Check sheet for the modelled part. Datum: model origin and axes. Units: mm. A direction names the side the tool comes from. Give positions to 0.01 mm unless a question says otherwise; leave off trailing zeros. Write each loop counter-clockwise with the first axis right and the second up, starting at its lowest first coordinate (ties: lowest second). Pieces come first, ordered by that corner, then holes. Notation, with made-up numbers: (-9, -36.75) -> (37, -36.75) arc R19 cw to (37, -11.75) -> close; hole circle Ø11 at (-32.5, 21.25). An arc over 180 degrees is marked (long way). Use a Markdown table: item, result. Add a question column.
1. Cross-section at D-D (z = 27). Enter the section's corners in (x, y), then the cut area to 3 significant figures.
2. Cross-section at B-B (z = 54). Enter the section's corners in (x, y), then the cut area to 3 significant figures.
3. Release check for a two-part mould opening along X. For faces 1 (the cylindrical face through (12.675, 34.614, 48.128)), 2 (the flat face through (180, 30, 12)), 3 (the cylindrical face through (52.017, 30.791, 12.675)) record: released by +X, released by -X, zero draft, split by the parting line, or undercut.
4. Cross-section at A-A (x = 70). Enter the section's corners in (y, z), then the cut area to 3 significant figures.
5. Cross-section at C-C (y = 26). Enter the section's corners in (x, z), then the cut area to 3 significant figures.
6. Set-up check for faces 4 (the flat face through (101, 30, 25)), 5 (the cylindrical face through (12.675, 8.555, 77.979)): record each of +Z, -Z, +X, -X, +Y, -Y from which the full face is reachable in a straight line by a thin tool's end or side.
7. Gauge pin test, flat ends, axial feed: P1, Ø3, axis at y = 31.5, z = 43, coming from the +X side; P2, Ø5, axis at x = 33.5, y = 9.5, coming from the +Z side; P3, Ø10, axis at x = 150.5, y = 14, coming from the -Z side. Record the tip position at first contact, or that the pin passes through.
8. Scan lines: probe 1 along Y at (x, z) = (135, 7.25); probe 2 along X at (y, z) = (19, 8.5); probe 3 along X at (y, z) = (41.5, 57). Record each from-to range of solid material in increasing order. Write a range as [from, to].
from build123d import *

# Parameters (mm, degrees)
F0_W      = 180
F0_H      = 60
F1_DEPTH  = 25
F2_W      = 25
F2_H      = 60
F3_DEPTH  = 62
F4_R      = 30
F5_R      = 29.99999
F6_R      = 18
F7_DEPTH  = 25
F8_SIZE   = 15
F9_R      = 10
F10_DEPTH = 25.001


# Not quite as in the source:
# - a fillet or chamfer is up to 0.001 mm smaller than in the source, because OpenCascade refuses the exact size


with BuildPart() as f1:
    # F0 (on Top) → F1 (new body)
    with BuildSketch(Plane.XY):
        with Locations((90, 30)):
            Rectangle(F0_W, F0_H)
    extrude(amount=F1_DEPTH)

    # F2 (on face) → F3 (join)
    with BuildSketch(Plane.XY.offset(25)):
        with Locations((12.5, 30)):
            Rectangle(F2_W, F2_H)
    extrude(amount=F3_DEPTH)

    # F4
    f4_edges = [f1.edges().sort_by_distance(p)[0] for p in [
        (12.5, 0, 87),
    ]]
    fillet(f4_edges, radius=F4_R)

    # F5 (radius 30 in the source; OpenCascade refuses exactly that, so slightly less here)
    f5_edges = [f1.edges().sort_by_distance(p)[0] for p in [
        (12.5, 60, 87),
    ]]
    fillet(f5_edges, radius=F5_R)

    # F6 (on face) → F7 (cut)
    with BuildSketch(Plane.XY.offset(25)):
        with Locations((70, 30)):
            Circle(F6_R)
        with Locations((135, 30)):
            Circle(F6_R)
    extrude(amount=-F7_DEPTH, mode=Mode.SUBTRACT)

    # F8
    f8_edges = [f1.edges().sort_by_distance(p)[0] for p in [
        (180, 0, 12.5),
        (180, 60, 12.5),
    ]]
    chamfer(f8_edges, length=F8_SIZE)

    # F9 (on face) → F10 (cut, through all)
    with BuildSketch(Plane.YZ.offset(25)):
        with Locations((30, 57)):
            Circle(F9_R)
    extrude(amount=-F10_DEPTH, mode=Mode.SUBTRACT)


solid = f1.part
Worked answers:
| question | item | result |
|---|---|---|
| 1 | outline | (0, 0) -> (25, 0) -> (25, 60) -> (0, 60) -> close |
| 1 | area | 1,500 mm² |
| 2 | outline | (0, 0) -> (25, 0) -> (25, 20.46) -> (0, 20.46) -> close; (0, 39.54) -> (25, 39.54) -> (25, 60) -> (0, 60) -> close |
| 2 | area | 1,020 mm² |
| 3 | face 1 | zero draft |
| 3 | face 2 | released by +X |
| 3 | face 3 | undercut |
| 4 | outline | (0, 0) -> (12, 0) -> (12, 25) -> (0, 25) -> close; (48, 0) -> (60, 0) -> (60, 25) -> (48, 25) -> close |
| 4 | area | 600 mm² |
| 5 | outline | (0, 0) -> (52.45, 0) -> (52.45, 25) -> (25, 25) -> (25, 47.83) -> (0, 47.83) -> close; (0, 66.17) -> (25, 66.17) -> (25, 86.73) -> (0, 86.73) -> close; (87.55, 0) -> (117.45, 0) -> (117.45, 25) -> (87.55, 25) -> close; (152.55, 0) -> (180, 0) -> (180, 25) -> (152.55, 25) -> close |
| 5 | area | 3,830 mm² |
| 6 | face 4 | +Z, +X, +Y, -Y |
| 6 | face 5 | +Z, +X, -X, -Y |
| 7 | P1 | stops at x = 25 |
| 7 | P2 | stops at z = 25 |
| 7 | P3 | stops at z = 0 |
| 8 | probe 1 | y = [0, 12], [48, 60] |
| 8 | probe 2 | x = [0, 55.75], [84.25, 120.75], [149.25, 180] |
| 8 | probe 3 | x = [0, 25] |
